```python
from build123d import *

# Parameters (mm, degrees)
F0_W     = 50.8
F0_H     = 12.7
F1_DEPTH = 3.175
F2_R     = 3.175
F3_DEPTH = 6.35
F5_DEPTH = 6.35
F6_R     = 6.34999
F7_R     = 3.175


# Not quite as in the source:
# - a fillet or chamfer is up to 0.001 mm smaller than in the source, because OpenCascade refuses the exact size


with BuildPart() as f1:
    # F0 (on Front) → F1 (new body)
    with BuildSketch(Plane.XZ):
        with Locations((25.4, 6.35)):
            Rectangle(F0_W, F0_H)
    extrude(amount=F1_DEPTH)

    # F2 (on face) → F3 (join)
    with BuildSketch(Plane(origin=(0, 0, 0), x_dir=(-1, 0, 0), z_dir=(0, 1, 0))):
        with Locations((-38.1, 6.35)):
            Circle(F2_R)
    extrude(amount=F3_DEPTH)

    # F4 (on face) → F5 (join)
    with BuildSketch(Plane.XZ.offset(3.175)):
        Polygon((25.4, 10.795), (25.4, 12.7), (0, 12.7), (0, 0), (25.4, 0), (25.4, 1.905), (1.905, 1.905), (1.905, 10.795), align=None)
    extrude(amount=F5_DEPTH)

    # F6 (radius 6.35 in the source; OpenCascade refuses exactly that, so slightly less here)
    f6_edges = [f1.edges().sort_by_distance(p)[0] for p in [
        (50.8, -1.5875, 0),
        (50.8, -1.5875, 12.7),
    ]]
    fillet(f6_edges, radius=F6_R)

    # F7
    f7_edges = [f1.edges().sort_by_distance(p)[0] for p in [
        (0, -4.7625, 12.7),
        (0, -4.7625, 0),
        (1.905, -6.35, 10.795),
        (1.905, -6.35, 1.905),
    ]]
    fillet(f7_edges, radius=F7_R)


solid = f1.part
```
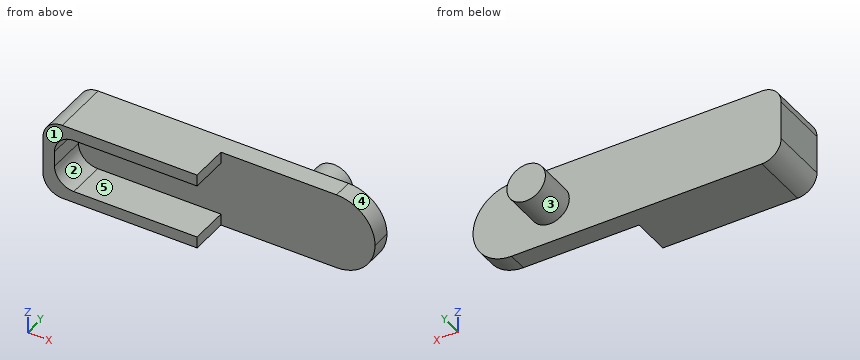
Can you work these out from the model? Positions are in its coordinate system, mm. Face numbers are marked on the shaded views. A direction names the side the tool comes from. Round coordinates to 2 decimals unless told otherwise and drop trailing zeros. Loops run counter-clockwise (first coordinate to the right, second up) from the corner with the lowest first, then second, coordinate; pieces in that order, holes last. Notation, with made-up numbers: M -34.5,41 L 6.5,41 A34 cw 6.5,76 Z; hole C 83,-25 d1. An arc over 180 degrees is marked long. Write item = value, one per line. Start each with the question number.
(1) Suppose I cut it at C-C on z = 4.5. Write out the boundary of the cut face in (x, y) (3 decimals).
(2) If we mould it in two halves opening along Z, with no side actions, what happens to the marked faces 1, 2 and 3? For each: released by +Z, released by -Z, zero draft, split by the parting line, or undercut.
(3) Suppose I cut it at B-B on y = -5.75. Write out the boundary of the cut face in (x, z) (3 decimals).
(4) I'm going to push flat-ended pins straight in: P1, Ø3, axis at y = -5.5, z = 7, coming from the +X side; P2, Ø1, axis at y = -6, z = 0.5, coming from the +X side; P3, Ø2, axis at y = -7, z = 11, coming from the -X side. Where does each tip first touch, or does it pass through?
(5) Suppose I cut it at A-A on x = 9. Write out the boundary of the cut face in (y, z) (3 decimals), plus the area to 3 significant figures.
(6) I need wall thicknesses on line 1 along Z through (x, y) = (12, -4.75) (3 decimals); line 2 along Y through (x, z) = (20, 1.75) (3 decimals); line 3 along Y through (x, z) = (18.5, 8.5) (3 decimals). Which ranges of each line are inside material? Lowest first, please.
(7) Suppose I cut it at D-D on x = 38.1. Write out the boundary of the cut face in (y, z) (3 decimals), plus the area to 3 significant figures.
(8) Which directions (+Z, -Z, +X, -X, +Y, -Y) give clear straight access to the entire face, cutting with the end or side of a thin tool? Please do the marked faces 4 and 5.
Answer block:
q1.outline = M 0,-9.525 L 1.958,-9.525 L 1.958,-3.175 L 50.525,-3.175 L 50.525,0 L 40.68,0 L 40.68,6.35 L 35.52,6.35 L 35.52,0 L 0,0 Z
q2.face_1 = zero draft
q2.face_2 = undercut
q2.face_3 = split by the parting line
q3.outline = M 0,3.175 A3.175 ccw 3.175,0 L 25.4,0 L 25.4,1.905 L 5.08,1.905 A3.175 cw 1.905,5.08 L 1.905,7.62 A3.175 cw 5.08,10.795 L 25.4,10.795 L 25.4,12.7 L 3.175,12.7 A3.175 ccw 0,9.525 Z
q4.P1 = 2.03
q4.P2 = 25.4
q4.P3 = 0.04
q5.outline = M -9.525,0 L 0,0 L 0,12.7 L -9.525,12.7 L -9.525,10.795 L -3.175,10.795 L -3.175,1.905 L -9.525,1.905 Z
q5.area = 64.5 mm²
q6.line_1 = 0 to 1.905, 10.795 to 12.7
q6.line_2 = -9.525 to 0
q6.line_3 = -3.175 to 0
q7.outline = M -3.175,0 L 0,0 L 0,3.175 L 6.35,3.175 L 6.35,9.525 L 0,9.525 L 0,12.7 L -3.175,12.7 Z
q7.area = 80.6 mm²
q8.face_4 = +Z, +X, +Y, -Y
q8.face_5 = +X, -Y
